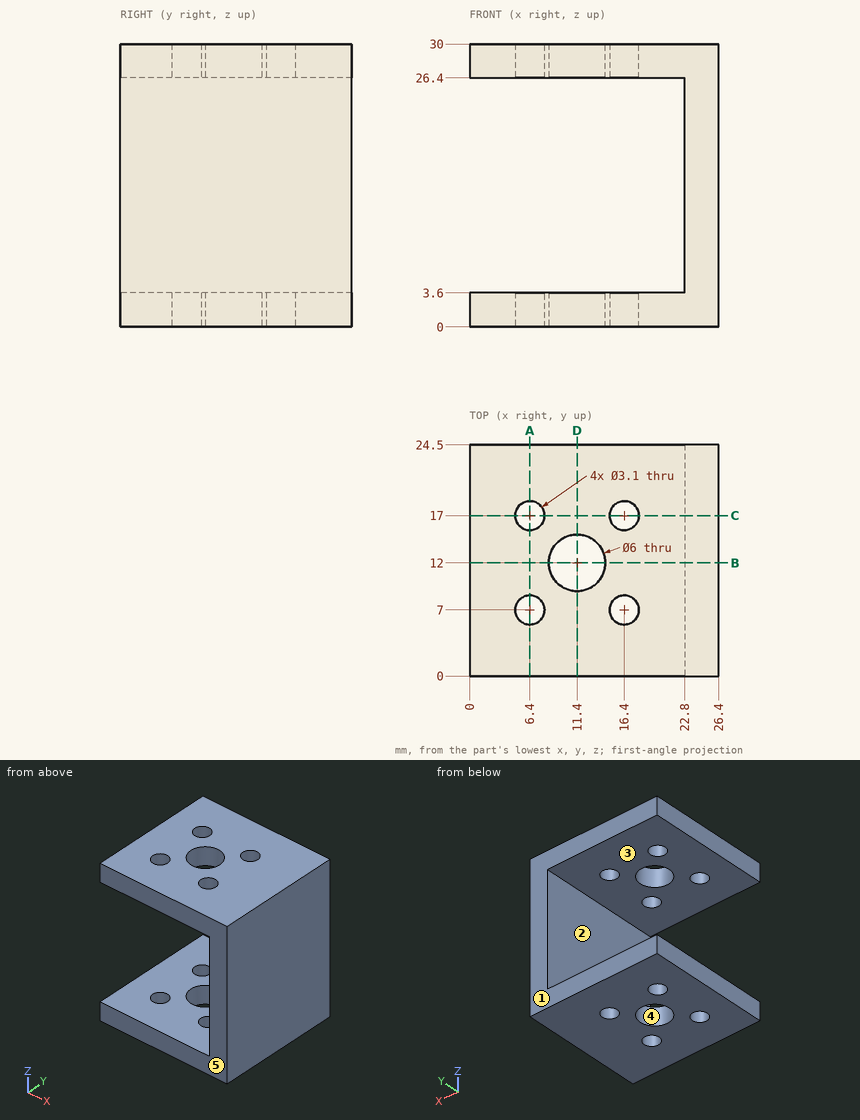
Design review of the part shown in the three views and the two pictorial views. Dimensions are in mm from the part's minimum x, y and z. A direction names the side the tool comes from. Give positions to 0.01 mm unless a question says otherwise; leave off trailing zeros. Write each loop counter-clockwise with the first axis right and the second up, starting at its lowest first coordinate (ties: lowest second). Pieces come first, ordered by that corner, then holes. Notation, with made-up numbers: M 29,-1.5 L 46,-1.5 A19 ccw 46,20.5 Z; hole C -11,-10.75 d6. An arc over 180 degrees is marked long. Answer in a Markdown table with one row per item.
Item 1: For P1, Ø10, axis at y = 4.5, z = 9, coming from the -X side; P2, Ø3.5, axis at x = 16.4, y = 17, coming from the -Z side; P3, Ø5, axis at x = 11.4, y = 12, coming from the -Z side, all flat-tipped, find the tip position at first contact; note any pin that passes through.
Check sheet entries:
| item | result |
|---|---|
| P1 | x = 22.8 |
| P2 | z = 0 |
| P3 | through |
Item 2: Add section D-D on x = 11.4. Give the boundary of the cut face in (y, z), plus the area to 3 significant figures.
Check sheet entries:
| item | result |
|---|---|
| outline | M 0,0 L 9,0 L 9,3.6 L 0,3.6 Z; M 0,26.4 L 9,26.4 L 9,30 L 0,30 Z; M 15,0 L 24.5,0 L 24.5,3.6 L 15,3.6 Z; M 15,26.4 L 24.5,26.4 L 24.5,30 L 15,30 Z |
| area | 133 mm2 |
Item 3: Add section B-B on y = 12. Give the boundary of the cut face in (x, z), plus the area to 3 significant figures.
Check sheet entries:
| item | result |
|---|---|
| outline | M 0,0 L 8.4,0 L 8.4,3.6 L 0,3.6 Z; M 0,26.4 L 8.4,26.4 L 8.4,30 L 0,30 Z; M 14.4,0 L 26.4,0 L 26.4,30 L 14.4,30 L 14.4,26.4 L 22.8,26.4 L 22.8,3.6 L 14.4,3.6 Z |
| area | 229 mm2 |
Item 4: Draft analysis for pull direction Y (two halves, no side actions). For the marked faces 3, 4 and 5, state which applies: +Y half, -Y half, draft (parallel to the pull), parting line (faces both ways), or undercut.
Check sheet entries:
| item | result |
|---|---|
| face 3 | draft |
| face 4 | undercut |
| face 5 | -Y half |
Item 5: Tool access review of the marked faces 1 and 2: name each direction out of +Z, -Z, +X, -X, +Y, -Y from which nothing blocks a thin tool from reaching the whole face with its end or side.
Check sheet entries:
| item | result |
|---|---|
| face 1 | +Z, -Z, +X, -X, +Y |
| face 2 | -X, +Y, -Y |
Item 6: For line 1 along Y through (x, z) = (16.4, 0.9); line 2 along X through (y, z) = (7, 28.7); line 3 along Z through (x, y) = (22.5, 13.25), list the stretches that pass through material, from the lowest coordinate up.
Check sheet entries:
| item | result |
|---|---|
| line 1 | 0 to 5.45, 8.55 to 15.45, 18.55 to 24.5 |
| line 2 | 0 to 4.85, 7.95 to 14.85, 17.95 to 26.4 |
| line 3 | 0 to 3.6, 26.4 to 30 |
Item 7: Add section A-A on x = 6.4. Give the boundary of the cut face in (y, z).
Check sheet entries:
| item | result |
|---|---|
| outline | M 0,0 L 5.45,0 L 5.45,3.6 L 0,3.6 Z; M 0,26.4 L 5.45,26.4 L 5.45,30 L 0,30 Z; M 8.55,0 L 15.45,0 L 15.45,3.6 L 8.55,3.6 Z; M 8.55,26.4 L 15.45,26.4 L 15.45,30 L 8.55,30 Z; M 18.55,0 L 24.5,0 L 24.5,3.6 L 18.55,3.6 Z; M 18.55,26.4 L 24.5,26.4 L 24.5,30 L 18.55,30 Z |
Item 8: Add section C-C on y = 17. Give the boundary of the cut face in (x, z), plus the area to 3 significant figures.
Check sheet entries:
| item | result |
|---|---|
| outline | M 0,0 L 4.85,0 L 4.85,3.6 L 0,3.6 Z; M 0,26.4 L 4.85,26.4 L 4.85,30 L 0,30 Z; M 7.95,0 L 14.85,0 L 14.85,3.6 L 7.95,3.6 Z; M 7.95,26.4 L 14.85,26.4 L 14.85,30 L 7.95,30 Z; M 17.95,0 L 26.4,0 L 26.4,30 L 17.95,30 L 17.95,26.4 L 22.8,26.4 L 22.8,3.6 L 17.95,3.6 Z |
| area | 228 mm2 |
